Input: part model. Units: mm. Frame: model coordinates. Face numbers are marked on the shaded views. A direction names the side the tool comes from. Give positions to 0.01 mm unless a question says otherwise; leave off trailing zeros. Order: outer loops, then holes, each group sorted by start corner. A loop starts at its lowest first (then second) coordinate and runs counter-clockwise, first axis right, second up. Notation, with made-up numbers: (69, -10) - (101, -10) arc R20 cw to (101, 9) - close; hole circle Ø8 at (65.25, 82). An arc over 180 degrees is marked (long way). Use a Markdown table: item, result.
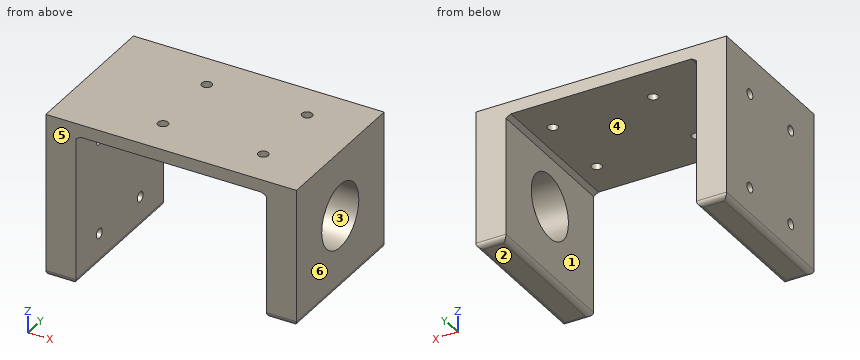
from build123d import *

# Parameters (mm, degrees)
SKETCH2_W                        = 127
SKETCH2_H                        = 76.2
BOSS_EXTRUDE1_DEPTH              = 6.35
F_13_64_0_20313_DIAMETER_HOLE1_D = 5.159502
SKETCH5_W                        = 15.24
SKETCH5_H                        = 76.2
BOSS_EXTRUDE2_DEPTH              = 63.5
CHAMFER1_SIZE                    = 2.54
CHAMFER1_SIZE2                   = 1.466469684
FILLET3_R                        = 2.54
SKETCH9_W                        = 15.24
SKETCH9_H                        = 76.2
BOSS_EXTRUDE3_DEPTH              = 76.2
CHAMFER5_SIZE                    = 2.54
CHAMFER5_SIZE2                   = 1.466469684
FILLET5_R                        = 2.54
CUT_EXTRUDE1_REACH               = 129
SKETCH17_R                       = 2.54
CUT_EXTRUDE2_REACH               = 129
SKETCH18_R                       = 16.129


with BuildPart() as part:
    # Sketch2 → Boss-Extrude1 (new body)
    with BuildSketch(Plane.XY):
        with Locations((-63.5, 38.1)):
            Rectangle(SKETCH2_W, SKETCH2_H)
    extrude(amount=BOSS_EXTRUDE1_DEPTH)

    # 13/64 (0.20313) Diameter Hole1 (through all)
    with Locations(Plane.XY.offset(6.35)):
        with Locations((-78.74, 57.15), (-78.74, 19.05), (-27.94, 57.15), (-27.94, 19.05)):
            Hole(F_13_64_0_20313_DIAMETER_HOLE1_D / 2)

    # Sketch5 → Boss-Extrude2 (add)
    with BuildSketch(Plane(origin=(0, 0, 0), x_dir=(-1, 0, 0), z_dir=(0, 0, -1))):
        with Locations((7.62, 38.1)):
            Rectangle(SKETCH5_W, SKETCH5_H)
    extrude(amount=BOSS_EXTRUDE2_DEPTH)

    # Chamfer1
    chamfer1_edges = [part.edges().sort_by_distance(p)[0] for p in [
        (-15.24, 38.1, 0),
    ]]
    chamfer1_side = [part.faces().sort_by_distance(p)[0] for p in [
        (-71.296336335, 38.1, 0),
    ]]
    chamfer(chamfer1_edges, length=CHAMFER1_SIZE, length2=CHAMFER1_SIZE2, reference=chamfer1_side[0])

    # Fillet3
    fillet3_edges = [part.edges().sort_by_distance(p)[0] for p in [
        (-15.24, 38.1, -63.5),
        (-7.62, 76.2, -63.5),
        (0, 38.1, -63.5),
        (-7.62, 0, -63.5),
    ]]
    fillet(fillet3_edges, radius=FILLET3_R)

    # Sketch9 → Boss-Extrude3 (add)
    with BuildSketch(Plane(origin=(0, 0, 0), x_dir=(-1, 0, 0), z_dir=(0, 0, -1))):
        with Locations((119.38, 38.1)):
            Rectangle(SKETCH9_W, SKETCH9_H)
    extrude(amount=BOSS_EXTRUDE3_DEPTH)

    # Chamfer5
    chamfer5_edges = [part.edges().sort_by_distance(p)[0] for p in [
        (-111.76, 38.1, 0),
    ]]
    chamfer5_side = [part.faces().sort_by_distance(p)[0] for p in [
        (-64.905058797, 38.1, 0),
    ]]
    chamfer(chamfer5_edges, length=CHAMFER5_SIZE, length2=CHAMFER5_SIZE2, reference=chamfer5_side[0])

    # Fillet5
    fillet5_edges = [part.edges().sort_by_distance(p)[0] for p in [
        (-127, 38.1, -76.2),
        (-119.38, 76.2, -76.2),
        (-111.76, 38.1, -76.2),
        (-119.38, 0, -76.2),
    ]]
    fillet(fillet5_edges, radius=FILLET5_R)

    # Sketch17 → Cut-Extrude1 (cut, up to next)
    with BuildSketch(Plane.ZY.offset(127), mode=Mode.PRIVATE) as cut_extrude1_sk1:
        with Locations((-12.7, 20.32)):
            Circle(SKETCH17_R)
    cut_extrude1_tool1 = extrude(cut_extrude1_sk1.sketch, amount=-CUT_EXTRUDE1_REACH, mode=Mode.PRIVATE) & part.part
    add(cut_extrude1_tool1.solids().sort_by_distance((-127, 20.32, -12.7))[0], mode=Mode.SUBTRACT)
    # Sketch17 → Cut-Extrude1 (cut, up to next)
    with BuildSketch(Plane.ZY.offset(127), mode=Mode.PRIVATE) as cut_extrude1_sk2:
        with Locations((-12.7, 55.88)):
            Circle(SKETCH17_R)
    cut_extrude1_tool2 = extrude(cut_extrude1_sk2.sketch, amount=-CUT_EXTRUDE1_REACH, mode=Mode.PRIVATE) & part.part
    add(cut_extrude1_tool2.solids().sort_by_distance((-127, 55.88, -12.7))[0], mode=Mode.SUBTRACT)
    # Sketch17 → Cut-Extrude1 (cut, up to next)
    with BuildSketch(Plane.ZY.offset(127), mode=Mode.PRIVATE) as cut_extrude1_sk3:
        with Locations((-60.7, 20.32)):
            Circle(SKETCH17_R)
    cut_extrude1_tool3 = extrude(cut_extrude1_sk3.sketch, amount=-CUT_EXTRUDE1_REACH, mode=Mode.PRIVATE) & part.part
    add(cut_extrude1_tool3.solids().sort_by_distance((-127, 20.32, -60.7))[0], mode=Mode.SUBTRACT)
    # Sketch17 → Cut-Extrude1 (cut, up to next)
    with BuildSketch(Plane.ZY.offset(127), mode=Mode.PRIVATE) as cut_extrude1_sk4:
        with Locations((-60.7, 55.88)):
            Circle(SKETCH17_R)
    cut_extrude1_tool4 = extrude(cut_extrude1_sk4.sketch, amount=-CUT_EXTRUDE1_REACH, mode=Mode.PRIVATE) & part.part
    add(cut_extrude1_tool4.solids().sort_by_distance((-127, 55.88, -60.7))[0], mode=Mode.SUBTRACT)

    # Sketch18 → Cut-Extrude2 (cut, up to next)
    with BuildSketch(Plane(origin=(0, 0, 0), x_dir=(0, 0, -1), z_dir=(1, 0, 0)), mode=Mode.PRIVATE) as cut_extrude2_sk1:
        with Locations((26.7, 38.02)):
            Circle(SKETCH18_R)
    cut_extrude2_tool1 = extrude(cut_extrude2_sk1.sketch, amount=-CUT_EXTRUDE2_REACH, mode=Mode.PRIVATE) & part.part
    add(cut_extrude2_tool1.solids().sort_by_distance((0, 38.02, -26.7))[0], mode=Mode.SUBTRACT)


solid = part.part
1. Set-up query: the marked faces 1, 2 and 3. Return all of +Z, -Z, +X, -X, +Y, -Y with unobstructed straight access to the full face (end or side cutting, diameter ignored); none if empty.
Response:
| item | result |
|---|---|
| face 1 | -Z, +Y, -Y |
| face 2 | -Z, +X, +Y, -Y |
| face 3 | +X |
2. Section query A-A (y = 38.02). Return loops of the section in (x, z).
Response:
| item | result |
|---|---|
| outline | (-127, -73.66) arc R2.54 ccw to (-124.46, -76.2) - (-114.3, -76.2) arc R2.54 ccw to (-111.76, -73.66) - (-111.76, -1.47) - (-109.22, 0) - (-17.78, 0) - (-15.24, -1.47) - (-15.24, -10.57) - (0, -10.57) - (0, 6.35) - (-127, 6.35) - close; (-15.24, -60.96) arc R2.54 ccw to (-12.7, -63.5) - (-2.54, -63.5) arc R2.54 ccw to (0, -60.96) - (0, -42.83) - (-15.24, -42.83) - close |
3. Mould query, pull axis X, two halves, no side actions, for the marked faces 4, 5 and 6. Classes: pulls with the +X half, pulls with the -X half, needs draft (parallel to the pull), parting line crosses it, or undercut.
Response:
| item | result |
|---|---|
| face 4 | undercut |
| face 5 | needs draft |
| face 6 | pulls with the +X half |
4. Pin query (flat end, axial travel): pin 1 (4 mm diameter, centred on y = 20.32, z = -60.7, fed in from -X); pin 2 (1.5 mm diameter, centred on x = -30.5, y = 9, fed in from -Z); pin 3 (8 mm diameter, centred on x = -9, y = 45, fed in from -Z). Return the tip coordinate at first contact, or that it passes through.
Response:
| item | result |
|---|---|
| pin 1 | stops at x = -15.24 |
| pin 2 | stops at z = 0 |
| pin 3 | stops at z = -63.5 |
5. Section query B-B (z = -50.5). Return loops of the section in (x, y), then the cut area to 3 significant figures.
Response:
| item | result |
|---|---|
| outline | (-127, 0) - (-111.76, 0) - (-111.76, 76.2) - (-127, 76.2) - close; (-15.24, 0) - (0, 0) - (0, 76.2) - (-15.24, 76.2) - close |
| area | 2,320 mm^2 |
6. Section query C-C (x = -78.74). Return loops of the section in (y, z), then the cut area to 3 significant figures.
Response:
| item | result |
|---|---|
| outline | (0, 0) - (16.47, 0) - (16.47, 6.35) - (0, 6.35) - close; (21.63, 0) - (54.57, 0) - (54.57, 6.35) - (21.63, 6.35) - close; (59.73, 0) - (76.2, 0) - (76.2, 6.35) - (59.73, 6.35) - close |
| area | 418 mm^2 |
7. Material intervals for line 1 along Y through (x, z) = (-27.94, 2.5); line 2 along X through (y, z) = (19, 1); line 3 along Y through (x, z) = (-117, -12.7), sorted ascending.
Response:
| item | result |
|---|---|
| line 1 | y = 0 to 16.47, 21.63 to 54.57, 59.73 to 76.2 |
| line 2 | x = -127 to -81.32, -76.16 to -30.52, -25.36 to 0 |
| line 3 | y = 0 to 17.78, 22.86 to 53.34, 58.42 to 76.2 |
8. Section query D-D (z = -12.7). Return loops of the section in (x, y).
Response:
| item | result |
|---|---|
| outline | (-127, 0) - (-111.76, 0) - (-111.76, 17.78) - (-127, 17.78) - close; (-127, 22.86) - (-111.76, 22.86) - (-111.76, 53.34) - (-127, 53.34) - close; (-127, 58.42) - (-111.76, 58.42) - (-111.76, 76.2) - (-127, 76.2) - close; (-15.24, 0) - (0, 0) - (0, 30.01) - (-15.24, 30.01) - close; (-15.24, 46.03) - (0, 46.03) - (0, 76.2) - (-15.24, 76.2) - close |
